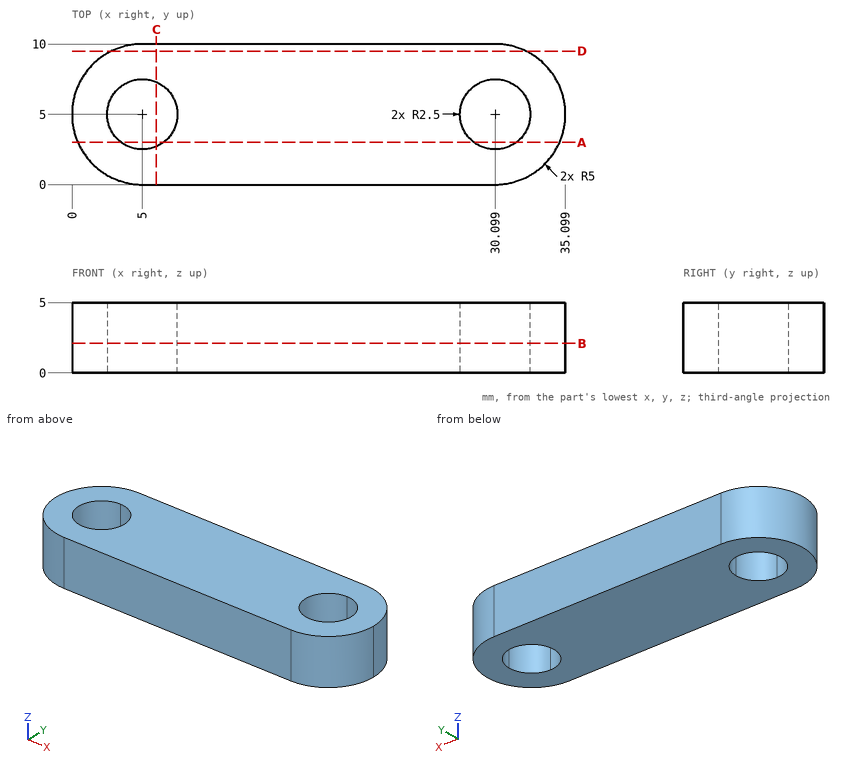
Can you work these out from the drawing? Everything is in mm from the part's minimum corner. Round coordinates to 2 decimals unless told otherwise and drop trailing zeros. Loops run counter-clockwise (first coordinate to the right, second up) from the corner with the lowest first, then second, coordinate; pieces in that order, holes last. Notation, with made-up numbers: (18, -17) - (66, -17) arc R34 ccw to (66, 18) - close; hole circle Ø10 at (-22, 21). An arc over 180 degrees is marked (long way). One line per question, with ' | ' between items. Start each with the question number.
Q1. I want a section at D-D (y = 9.5). Write out the boundary of the cut face in (x, z).
Q2. I want a section at A-A (y = 3). Write out the boundary of the cut face in (x, z), then the cut area to 3 significant figures.
Q3. I want a section at C-C (x = 6). Write out the boundary of the cut face in (y, z).
Q4. I want a section at B-B (z = 2.1). Write out the boundary of the cut face in (x, y), then the cut area to 3 significant figures.
Q5. Please list where these lines run through material, in increasing order: line 1 (X direction, y = 2.75, z = 1.2) (1 decimal); line 2 (Y direction, x = 5, z = 2.45); line 3 (X direction, y = 3, z = 0.3). Write a range as [from, to].
Q6. Will these pins go through, and if not, where does the flat tip stop? pin 1 (4 mm diameter, centred on x = 14.5, y = 7, fed in from -Z); pin 2 (1.5 mm diameter, centred on y = 7.5, z = 1.5, fed in from +X); pin 3 (1 mm diameter, centred on y = 8, z = 4, fed in from -X); pin 4 (2 mm diameter, centred on y = 7, z = 0.5, fed in from -X).
Response values:
1) outline: (2.82, 0) - (32.28, 0) - (32.28, 5) - (2.82, 5) - close
2) outline: (0.42, 0) - (3.5, 0) - (3.5, 5) - (0.42, 5) - close; (6.5, 0) - (28.6, 0) - (28.6, 5) - (6.5, 5) - close; (31.6, 0) - (34.68, 0) - (34.68, 5) - (31.6, 5) - close | area: 141 mm²
3) outline: (0, 0) - (2.71, 0) - (2.71, 5) - (0, 5) - close; (7.29, 0) - (10, 0) - (10, 5) - (7.29, 5) - close
4) outline: (5, 0) - (30.1, 0) arc R5 ccw to (30.1, 10) - (5, 10) arc R5 ccw to start; hole circle Ø5 at (5, 5); hole circle Ø5 at (30.1, 5) | area: 290 mm²
5) line 1: x = [0.5, 3.9], [6.1, 29], [31.2, 34.6] | line 2: y = [0, 2.5], [7.5, 10] | line 3: x = [0.42, 3.5], [6.5, 28.6], [31.6, 34.68]
6) pin 1: stops at z = 0 | pin 2: stops at x = 34.78 | pin 3: stops at x = 0.67 | pin 4: stops at x = 0.1
